Source: three-view drawing plus pictorial views. Frame: mm from the lowest corner of the part. Give positions to 0.01 mm unless a question says otherwise; leave off trailing zeros. Loops run counter-clockwise (first coordinate to the right, second up) from the corner with the lowest first, then second, coordinate; pieces in that order, holes last.
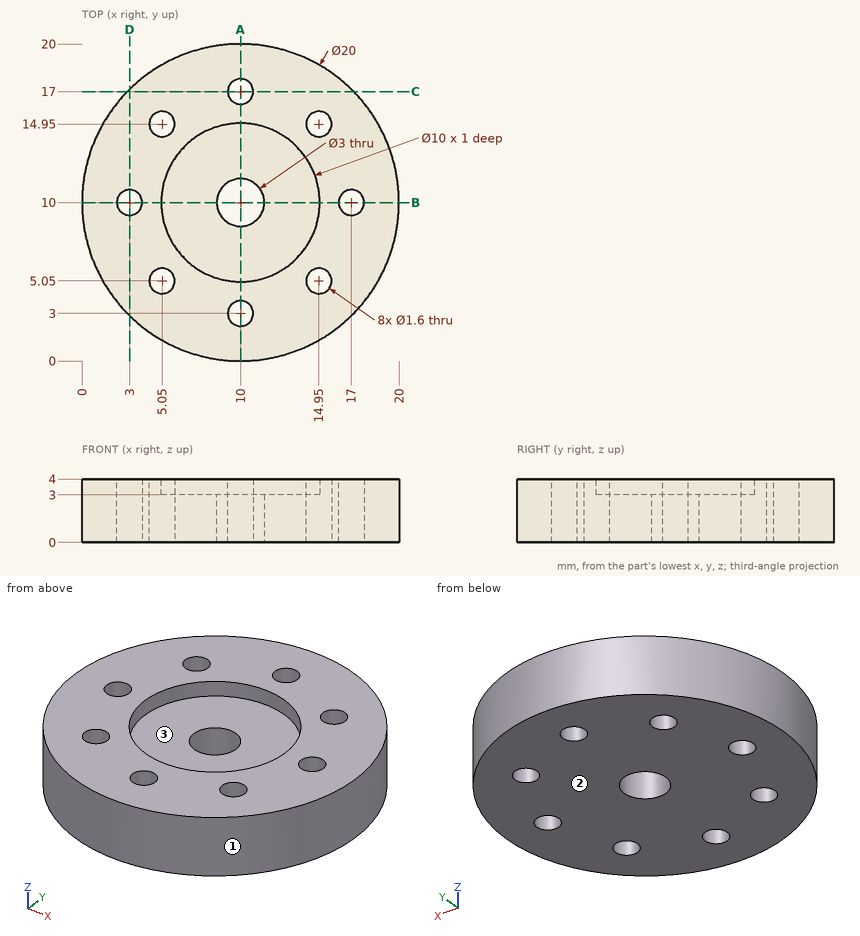
Q1. Mould query, pull axis X, two halves, no side actions, for the marked faces 1, 2 and 3. Classes: +X half, -X half, draft (parallel to the pull), parting line (faces both ways), or undercut.
Q2. Section query A-A, the plane x = 10. Return loops of the section in (y, z).
Q3. Material intervals for probe 1 along Y at (x, z) = (10, 1.85); probe 2 along Y at (x, z) = (5.5, 2.35); probe 3 along X at (y, z) = (10.5, 1.2) (1 decimal), sorted ascending.
Q4. Pin query (flat end, axial travel): pin 1 Ø1.5 at (y, z) = (14, 2) entering from -X; pin 2 Ø3 at (x, y) = (11, 9) entering from +Z. Return the tip coordinate at first contact, or that it passes through.
Q5. Section query C-C, the plane y = 17. Return loops of the section in (x, z).
Resolved:
1. face 1: parting line
1. face 2: draft
1. face 3: undercut
2. outline: (0, 0) - (2.2, 0) - (2.2, 4) - (0, 4) - close; (3.8, 0) - (8.5, 0) - (8.5, 3) - (5, 3) - (5, 4) - (3.8, 4) - close; (11.5, 0) - (16.2, 0) - (16.2, 4) - (15, 4) - (15, 3) - (11.5, 3) - close; (17.8, 0) - (20, 0) - (20, 4) - (17.8, 4) - close
3. probe 1: y = 0 to 2.2, 3.8 to 8.5, 11.5 to 16.2, 17.8 to 20
3. probe 2: y = 1.07 to 4.39, 5.71 to 14.29, 15.61 to 18.93
3. probe 3: x = 0 to 2.4, 3.6 to 8.6, 11.4 to 16.4, 17.6 to 20
4. pin 1: stops at x = 0.54
4. pin 2: stops at z = 3
5. outline: (2.86, 0) - (9.2, 0) - (9.2, 4) - (2.86, 4) - close; (10.8, 0) - (17.14, 0) - (17.14, 4) - (10.8, 4) - close
